Autodesk Inventor part; units mm, degrees
ref_plane "YZ Plane" through (0, 0, 0) normal (1, 0, 0) x (0, 1, 0)
ref_plane "XZ Plane" through (0, 0, 0) normal (0, 1, 0) x (-1, 0, 0)
ref_plane "XY Plane" through (0, 0, 0) normal (0, 0, 1) x (1, 0, 0)
sketch "Esquisse1" plane through (0, 0, 0) normal (0, 1, 0) x (-1, 0, 0)
  circle A0 centre (0, 0) radius 6.95
  circle A1 centre (0, 0) radius 5
  dimension "d0" = 13.9
  dimension "d1" = 10
extrude "Extrusion1" add sketch "Esquisse1" along normal blind 1.5
sketch "Esquisse2" plane through (0, 1.5, 0) normal (0, 1, 0) x (1, 0, 0)
  circle A0 centre (0, 0) radius 5
  circle A1 centre (0, 0) radius 5.95
  dimension "d4" = 11.9
extrude "Extrusion2" add sketch "Esquisse2" along normal blind 1.5
sketch "Esquisse3" plane through (0, 3, 0) normal (0, 1, 0) x (1, 0, 0)
  circle A0 centre (0, 0) radius 2.25
  circle A1 centre (0, 0) radius 5.95
  dimension "d7" = 4.5
extrude "Extrusion3" add sketch "Esquisse3" along normal blind 3
properties part number "moyeu_end"
Geometry check sheet. Reference: the model listing, model coordinates, mm. A direction names the side the tool comes from. Coordinates: 2 decimals unless noted, no trailing zeros. Write each loop counter-clockwise with the first axis right and the second up, starting at its lowest first coordinate (ties: lowest second). Pieces come first, ordered by that corner, then holes. Notation, with made-up numbers: M 80.25,-39.5 L 124.25,-39.5 A15 cw 124.25,-11.5 Z; hole C 69,88.5 d2. An arc over 180 degrees is marked long. One line per item, written item: value. Start each with the question number.
(1) Release check for a two-part mould opening along X. For faces 1 (the face through (-0.29, 4.48, 2.23)), 2 (the face through (2, 0, 5)), 3 (the face through (1.507, 0.74, 6.785)) record: released by +X, released by -X, zero draft, split by the parting line, or undercut.
(2) Scan lines: line 1 along Z through (x, y) = (0, 5.25); line 2 along Z through (x, y) = (0, 0.9). Record each from-to range of solid material in increasing order. Write a range as [from, to].
(3) Sectioned sample at C-C, the plane y = 0.45. Enter the section's corners in (x, z), and give its area (3 significant figures).
(4) Depth check by flat-ended pin: pin 1 (3 mm diameter, centred on x = 1.5, z = -2.5, fed in from -Y); pin 2 (2 mm diameter, centred on y = 4, z = -3, fed in from +X); pin 3 (2 mm diameter, centred on y = 1.5, z = -3.5, fed in from +X); pin 4 (3.5 mm diameter, centred on x = 0, z = 0, fed in from -Y). Enter the tip coordinate at first touch or a pass-through.
(5) Sectioned sample at B-B, the plane z = -4.25. Enter the section's corners in (x, y).
(6) Sectioned sample at D-D, the plane z = 5.5. Enter the section's corners in (x, y).
(7) Tool access check on faces 4 (the face through (-4.385, 3.718, 4.021)), 5 (the face through (3, 6, 0)), 6 (the face through (0, 2, 5)). Record the directions out of +Z, -Z, +X, -X, +Y, -Y that give a thin tool (end or side, any length) a straight path to the whole face; none if there is none.
Filled sheet:
1. face 1: undercut
1. face 2: zero draft
1. face 3: split by the parting line
2. line 1: [-5.95, -2.25], [2.25, 5.95]
2. line 2: [-6.95, -5], [5, 6.95]
3. outline: C 0,0 d13.9; hole C 0,0 d10
3. area: 73.2 mm²
4. pin 1: y = 3
4. pin 2: x = 5.6
4. pin 3: x = 6.48
4. pin 4: through
5. outline: M -5.5,0 L -2.63,0 L -2.63,3 L 2.63,3 L 2.63,0 L 5.5,0 L 5.5,1.5 L 4.16,1.5 L 4.16,6 L -4.16,6 L -4.16,1.5 L -5.5,1.5 Z
6. outline: M -4.25,0 L 4.25,0 L 4.25,1.5 L 2.27,1.5 L 2.27,6 L -2.27,6 L -2.27,1.5 L -4.25,1.5 Z
7. face 4: +Y
7. face 5: +Z, -Z, +X, -X, +Y
7. face 6: -Y
